Autodesk Inventor part; units mm, degrees
ref_plane "YZ Plane" through (0, 0, 0) normal (1, 0, 0) x (0, 1, 0)
ref_plane "XZ Plane" through (0, 0, 0) normal (0, 1, 0) x (-1, 0, 0)
ref_plane "XY Plane" through (0, 0, 0) normal (0, 0, 1) x (1, 0, 0)
sketch "Sketch1" plane through (0, 0, 0) normal (0, 1, 0) x (-1, 0, 0)
  line L0 (0, -4) -> (0, 5)
  line L1 (0, 5) -> (5, 5)
  line L2 (5, 5) -> (5, 11)
  line L3 (5, 11) -> (-6.5, 11)
  line L4 (-6.5, 11) -> (-6.5, 12.5)
  line L5 (-6.5, 12.5) -> (-10.634, 12.5)
  line L6 (-10.634, 12.5) -> (-11.5, 11)
  line L7 (-11.5, 11) -> (-11.5, -4)
  line L8 (-11.5, -4) -> (0, -4)
  line L9 (0, 0) -> (-4.5, 0) construction
  arc A0 (0, 5) -> (0, 2) centre (0, 3.5) ccw
  arc A1 (-6.5, 11) -> (-3.5, 11) centre (-5, 11) ccw
  dimension "d0" = 5
  dimension "d1" = 6
  dimension "d2" = 15
  dimension "d3" = 4.5
  dimension "d4" = 1.5
  dimension "d5" = 1.5
  dimension "d6" = 6.5
  dimension "d7" = 30
  dimension "d8" = 5
  dimension "d18" = 4
extrude "Extrusion1" add sketch "Sketch1" along normal mid plane 5 contours L8 L7 L6 L5 L4 A1 L3 L2 L1 A0 L0
sketch "Sketch2" plane through (0, -2.5, 2) normal (-1, 0, 0) x (0, 0, 1)
  point P0 (-2, 2.5)
  point P1 (-2, 2.5)
hole "Hole1" at (0, 0, 0) direction (1, 0, 0) diameter 2.459 end through all
properties part number "TorsoElectronicBoxLatchFrame" material "Acetal Resin, Black"
Source: CAD feature listing. Evaluate the final solid. Frame: model axes, mm. A direction names the side the tool comes from. Round coordinates to 2 decimals unless told otherwise and drop trailing zeros. Loops run counter-clockwise (first coordinate to the right, second up) from the corner with the lowest first, then second, coordinate; pieces in that order, holes last.
1. Section query A-A on z = 0. Output: boundary loops of the cut face in (x, y).
2. Section query D-D on y = -1.65. Output: boundary loops of the cut face in (x, z), and give its area (3 significant figures).
3. Contact query for flat-ended pins moving along their axis: pin 1 (1.2 mm diameter, centred on y = 0.5, z = 12, fed in from -X); pin 2 (2.5 mm diameter, centred on y = -0.5, z = -1, fed in from -X); pin 3 (1 mm diameter, centred on x = 3, y = 1.5, fed in from +Z). Output: stop coordinate, or through.
4. Mould query, pull axis Y, two halves, no side actions, for faces 4 (the cylindrical face through (5.83, 0.748, -0.976)), 5 (the flat face through (-2, 0, 5)), 6 (the flat face through (5, 2.5, 4)). Classes: released by +Y, released by -Y, zero draft, split by the parting line, or undercut.
5. Access query for faces 1 (the flat face through (-1, 0, 11)), 2 (the flat face through (9, 0, 12.5)), 3 (the flat face through (0, 0, -2)). Directions: +Z, -Z, +X, -X, +Y, -Y. A direction counts if a zero-diameter tool reaches every point of the face in a straight line with its end or side. Return the directions, or none.
6. Section query C-C on x = 5. Output: boundary loops of the cut face in (y, z).
7. Section query B-B on y = -0.3. Output: boundary loops of the cut face in (x, z).
8. Ray query, L1, parallel to Y at x = 8.5, z = 0; L2, parallel to Z at x = 3, y = 0; L3, parallel to Z at x = 1.25, y = 0.35. Return the intervals inside material, ascending.
Answers below:
1. outline: (0, -2.5) - (11.5, -2.5) - (11.5, -1.23) - (0, -1.23) - close; (0, 1.23) - (11.5, 1.23) - (11.5, 2.5) - (0, 2.5) - close
2. outline: (-5, 5) - (0, 5) arc R1.5 cw to (0, 2) - (0, -4) - (11.5, -4) - (11.5, 11) - (10.63, 12.5) - (6.5, 12.5) - (6.5, 11) arc R1.5 cw to (3.5, 11) - (-5, 11) - close
2. area: 202 mm2
3. pin 1: stops at x = 6.5
3. pin 2: stops at x = 0
3. pin 3: stops at z = 11
4. face 4: undercut
4. face 5: zero draft
4. face 6: released by +Y
5. face 1: +Z, -X, +Y, -Y
5. face 2: +Z, +X, -X, +Y, -Y
5. face 3: -Z, -X, +Y, -Y
6. outline: (-2.5, -4) - (2.5, -4) - (2.5, 9.5) - (-2.5, 9.5) - close; hole circle Ø2.46 at (0, 0)
7. outline: (-5, 5) - (0, 5) arc R1.5 cw to (0, 2) - (0, 1.19) - (11.5, 1.19) - (11.5, 11) - (10.63, 12.5) - (6.5, 12.5) - (6.5, 11) arc R1.5 cw to (3.5, 11) - (-5, 11) - close; (0, -4) - (11.5, -4) - (11.5, -1.19) - (0, -1.19) - close
8. L1: y = -2.5 to -1.23, 1.23 to 2.5
8. L2: z = -4 to -1.23, 1.23 to 11
8. L3: z = -4 to -1.18, 1.18 to 2.67, 4.33 to 11
